Geometry check sheet. Reference: the model listing, model coordinates, mm. A direction names the side the tool comes from. Round coordinates to 2 decimals unless told otherwise and drop trailing zeros. Write item = value, one per line.
Autodesk Fusion 360 part; units mm, degrees
sketch "Sketch1" plane through (0, 0, 0) normal (0, 1, 0) x (1, 0, 0)
  circle A0 centre (0, 0) radius 3.3909
  circle A1 centre (0, 0) radius 2.3368
  dimension "d1" = 6.7818
  dimension "d2" = 4.6736
extrude "Extrude1" add sketch "Sketch1" along normal blind 1.9304
sketch "Sketch2" plane through (0, 1.9304, 0) normal (0, 1, 0) x (-1, 0, 0)
  circle A0 centre (0, 0) radius 2.3368
  circle A1 centre (0, 0) radius 3.3909
  line L0 (-10.0076, 10.0076) -> (10.0076, 10.0076) construction
  line L1 (10.0076, 10.0076) -> (10.0076, -10.0076) construction
  line L2 (10.0076, -10.0076) -> (-10.0076, -10.0076) construction
  line L3 (-10.0076, -10.0076) -> (-10.0076, 10.0076) construction
  line L4 (-10.0076, 10.0076) -> (10.0076, -10.0076) construction
  line L5 (10.0076, 10.0076) -> (-10.0076, -10.0076) construction
  circle A2 centre (7.9709, -7.9709) radius 2.0367 construction
  circle A3 centre (-7.9709, -7.9709) radius 2.0367 construction
  circle A4 centre (-7.9709, 7.9709) radius 2.0367 construction
  circle A5 centre (7.9709, 7.9709) radius 2.0367 construction
  circle A6 centre (0, 0) radius 5.334 construction
  circle A7 centre (7.9709, -7.9709) radius 0.5
  circle A8 centre (-7.9709, -7.9709) radius 0.5
  circle A9 centre (7.9709, 7.9709) radius 0.5
  circle A10 centre (-7.9709, 7.9709) radius 0.5
  line L6 (8.4709, -7.9709) -> (-8.4709, -7.9709) construction
  line L7 (0, -5.334) -> (0, 5.334) construction
  line L8 (5.334, 0) -> (-5.334, 0) construction
  line L9 (9.4111, -6.5307) -> (6.5307, -9.4111) construction
  line L10 (-6.5307, -9.4111) -> (-9.4111, -6.5307) construction
  line L11 (-9.4111, 6.5307) -> (-6.5307, 9.4111) construction
  line L12 (9.4111, 6.5307) -> (6.5307, 9.4111) construction
  line L13 (5.334, 0) -> (9.6916, -6.8813)
  line L14 (5.334, 0) -> (9.6916, 6.8813)
  line L15 (0, 5.334) -> (6.8813, 9.6916)
  line L16 (0, 5.334) -> (-6.8813, 9.6916)
  line L17 (-5.334, 0) -> (-9.6916, 6.8813)
  line L18 (-5.334, 0) -> (-9.6916, -6.8813)
  line L19 (0, -5.334) -> (-6.8813, -9.6916)
  line L20 (0, -5.334) -> (6.8813, -9.6916)
  arc A11 (6.8813, -9.6916) -> (9.6916, -6.8813) centre (7.9709, -7.9709) ccw
  arc A12 (-9.6916, -6.8813) -> (-6.8813, -9.6916) centre (-7.9709, -7.9709) ccw
  arc A13 (-6.8813, 9.6916) -> (-9.6916, 6.8813) centre (-7.9709, 7.9709) ccw
  arc A14 (9.6916, 6.8813) -> (6.8813, 9.6916) centre (7.9709, 7.9709) ccw
  circle A15 centre (0, 0) radius 1.143
  dimension "d5" = 20.0152
  dimension "d6" = 20.0152
  dimension "d7" = 10.668
  dimension "d8" = 1
  dimension "d9" = 16.9418
  dimension "d10" = 2.286
extrude "Extrude2" add sketch "Sketch2" along normal blind 1.651 contours A0 | A1 | A7 | A8 | A9 | A10 | L13 L14 L15 L16 L17 L18 L19 L20 A11 A12 A13 A14
sketch "Sketch3" plane through (0, 3.5814, 0) normal (0, 1, 0) x (-1, 0, 0)
  circle A0 centre (0, 0) radius 1.143
  line L0 (5.334, 0) -> (9.6916, 6.8813)
  arc A1 (9.6916, 6.8813) -> (6.8813, 9.6916) centre (7.9709, 7.9709) ccw
  line L1 (6.8813, 9.6916) -> (0, 5.334)
  line L2 (0, 5.334) -> (-6.8813, 9.6916)
  arc A2 (-6.8813, 9.6916) -> (-9.6916, 6.8813) centre (-7.9709, 7.9709) ccw
  line L3 (-9.6916, 6.8813) -> (-5.334, 0)
  line L4 (-5.334, 0) -> (-9.6916, -6.8813)
  arc A3 (-9.6916, -6.8813) -> (-6.8813, -9.6916) centre (-7.9709, -7.9709) ccw
  line L5 (-6.8813, -9.6916) -> (0, -5.334)
  line L6 (0, -5.334) -> (6.8813, -9.6916)
  arc A4 (6.8813, -9.6916) -> (9.6916, -6.8813) centre (7.9709, -7.9709) ccw
  line L7 (9.6916, -6.8813) -> (5.334, 0)
  line L8 (-10.0076, 10.0076) -> (10.0076, 10.0076) construction
  line L9 (10.0076, 10.0076) -> (10.0076, -10.0076) construction
  line L10 (10.0076, -10.0076) -> (-10.0076, -10.0076) construction
  line L11 (-10.0076, -10.0076) -> (-10.0076, 10.0076) construction
  line L12 (-10.0076, 10.0076) -> (10.0076, -10.0076) construction
  line L13 (10.0076, 10.0076) -> (-10.0076, -10.0076) construction
  line L14 (8.2888, -8.2888) -> (-8.2888, 8.2888) construction
  line L15 (-8.2888, -8.2888) -> (8.2888, 8.2888) construction
  line L16 (-8.4455, 8.4455) -> (8.4455, 8.4455) construction
  line L17 (8.4455, 8.4455) -> (8.4455, -8.4455) construction
  line L18 (8.4455, -8.4455) -> (-8.4455, -8.4455) construction
  line L19 (-8.4455, -8.4455) -> (-8.4455, 8.4455) construction
  line L20 (-8.4455, 8.4455) -> (8.4455, -8.4455) construction
  line L21 (8.4455, 8.4455) -> (-8.4455, -8.4455) construction
  circle A5 centre (7.9104, -7.9104) radius 0.5351
  circle A6 centre (-7.9104, -7.9104) radius 0.5351
  circle A7 centre (-7.9104, 7.9104) radius 0.5351
  circle A8 centre (7.9104, 7.9104) radius 0.5351
  line L22 (-6.376, 6.376) -> (6.376, 6.376) construction
  line L23 (6.376, 6.376) -> (6.376, -6.376) construction
  line L24 (6.376, -6.376) -> (-6.376, -6.376) construction
  line L25 (-6.376, -6.376) -> (-6.376, 6.376) construction
  line L26 (-6.376, 6.376) -> (6.376, -6.376) construction
  line L27 (6.376, 6.376) -> (-6.376, -6.376) construction
  line L28 (-6.5278, 6.5278) -> (6.5278, 6.5278) construction
  line L29 (6.5278, 6.5278) -> (6.5278, -6.5278) construction
  line L30 (6.5278, -6.5278) -> (-6.5278, -6.5278) construction
  line L31 (-6.5278, -6.5278) -> (-6.5278, 6.5278) construction
  line L32 (-6.5278, 6.5278) -> (6.5278, -6.5278) construction
  line L33 (6.5278, 6.5278) -> (-6.5278, -6.5278) construction
  circle A9 centre (6.0095, -6.0095) radius 0.5183
  circle A10 centre (-6.0095, -6.0095) radius 0.5183
  circle A11 centre (-6.0095, 6.0095) radius 0.5183
  circle A12 centre (6.0095, 6.0095) radius 0.5183
  line L34 (-4.826, -4.826) -> (4.826, -4.826) construction
  line L35 (4.826, -4.826) -> (4.826, 4.826) construction
  line L36 (4.826, 4.826) -> (-4.826, 4.826) construction
  line L37 (-4.826, 4.826) -> (-4.826, -4.826) construction
  line L38 (-4.826, -4.826) -> (4.826, 4.826) construction
  line L39 (4.826, -4.826) -> (-4.826, 4.826) construction
  line L40 (-4.6338, -4.6338) -> (4.6338, -4.6338) construction
  line L41 (4.6338, -4.6338) -> (4.6338, 4.6338) construction
  line L42 (4.6338, 4.6338) -> (-4.6338, 4.6338) construction
  line L43 (-4.6338, 4.6338) -> (-4.6338, -4.6338) construction
  line L44 (-4.6338, -4.6338) -> (4.6338, 4.6338) construction
  line L45 (4.6338, -4.6338) -> (-4.6338, 4.6338) construction
  circle A13 centre (4.1698, -4.1698) radius 0.6562
  circle A14 centre (-4.1698, -4.1698) radius 0.6562
  circle A15 centre (-4.1698, 4.1698) radius 0.6562
  circle A16 centre (4.1698, 4.1698) radius 0.6562
  dimension "d13" = 23.4442
  dimension "d14" = 16.891
  dimension "d15" = 16.891
  dimension "d16" = 18.034
  dimension "d17" = 13.0556
  dimension "d18" = 13.1064
  dimension "d19" = 9.652
hole "Hole1" at (-7.9104, 3.5814, -7.9104) at (-6.0095, 3.5814, -6.0095) at (-4.1698, 3.5814, -4.1698) at (-7.9104, 3.5814, 7.9104) at (-6.0095, 3.5814, 6.0095) at (-4.1698, 3.5814, 4.1698) at (7.9104, 3.5814, 7.9104) at (6.0095, 3.5814, 6.0095) at (4.1698, 3.5814, 4.1698) at (7.9104, 3.5814, -7.9104) at (6.0095, 3.5814, -6.0095) at (4.1698, 3.5814, -4.1698) direction (0, -1, 0) diameter 1 end through all
sketch "Sketch4" plane through (0, 3.5814, 0) normal (0, 1, 0) x (-1, 0, 0)
  circle A0 centre (-6.0095, -6.0095) radius 0.5
  circle A1 centre (-4.1698, 4.1698) radius 0.5
  circle A2 centre (-7.9104, 7.9104) radius 0.5
  circle A3 centre (6.0095, 6.0095) radius 0.5
  circle A4 centre (4.1698, -4.1698) radius 0.5
  circle A5 centre (7.9104, -7.9104) radius 0.5
  circle A6 centre (6.0095, -6.0095) radius 0.5
  circle A7 centre (7.9104, 7.9104) radius 0.5
  circle A8 centre (4.1698, 4.1698) radius 0.5
  circle A9 centre (-6.0095, 6.0095) radius 0.5
  circle A10 centre (-7.9104, -7.9104) radius 0.5
  circle A11 centre (-4.1698, -4.1698) radius 0.5
  circle A12 centre (0, 0) radius 1.143
  line L0 (5.334, 0) -> (9.6916, 6.8813)
  arc A13 (9.6916, 6.8813) -> (6.8813, 9.6916) centre (7.9709, 7.9709) ccw
  line L1 (6.8813, 9.6916) -> (0, 5.334)
  line L2 (0, 5.334) -> (-6.8813, 9.6916)
  arc A14 (-6.8813, 9.6916) -> (-9.6916, 6.8813) centre (-7.9709, 7.9709) ccw
  line L3 (-9.6916, 6.8813) -> (-5.334, 0)
  line L4 (-5.334, 0) -> (-9.6916, -6.8813)
  arc A15 (-9.6916, -6.8813) -> (-6.8813, -9.6916) centre (-7.9709, -7.9709) ccw
  line L5 (-6.8813, -9.6916) -> (0, -5.334)
  line L6 (0, -5.334) -> (6.8813, -9.6916)
  arc A16 (6.8813, -9.6916) -> (9.6916, -6.8813) centre (7.9709, -7.9709) ccw
  line L7 (9.6916, -6.8813) -> (5.334, 0)
  circle A17 centre (0, 0) radius 2.7305
  circle A18 centre (0, 0) radius 2.2098
  dimension "d22" = 5.461
  dimension "d23" = 4.4196
extrude "Extrude3" add sketch "Sketch4" along normal blind 0.508 contours A17
extrude "Extrude4" cut 1 faces at (-1.8417, 3.5814, -0.1666) along direction (0, -1, 0) blind 1.016 from surface at -0.508
extrude "Extrude5" cut 1 faces at (1.9259, 1.9304, 0.1729) along direction (0, 1, 0) blind 2.0066 from surface at -1.9304
(1) Scan lines: L1, parallel to Z at x = 6.25, y = 2.85; L2, parallel to Z at x = 8, y = 3.1; L3, parallel to Y at x = -4.5, z = -2.75. Record each from-to range of solid material in increasing order. Write a range as [from, to].
Answers follow:
L1 = [-9.29, -6.45], [-5.57, -1.45], [1.45, 5.57], [6.45, 9.29]
L2 = [-10.01, -8.4], [-7.42, -4.21], [4.21, 7.42], [8.4, 10.01]
L3 = [1.93, 3.58]
(2) Set-up check for faces 4 (the cylindrical face through (-5.71, 2.74, 5.61)), 5 (the flat face through (-3.39, 2.74, -7.48)), 6 (the flat face through (-1, 3.073, -1)): record each of +Z, -Z, +X, -X, +Y, -Y from which the full face is reachable in a straight line by a thin tool's end or side.
Answers follow:
face_4 = +Y, -Y
face_5 = -Z, +Y, -Y
face_6 = +Y
(3) Gauge pin test, flat ends, axial feed: pin 1 (1.8 mm diameter, centred on x = 0, z = 0, fed in from -Y); pin 2 (3 mm diameter, centred on x = 3.5, z = 4, fed in from -Y); pin 3 (2 mm diameter, centred on x = 0, z = -4.5, fed in from +Y). Record the tip position at first contact, or that the pin passes through.
Answers follow:
pin_1 = through
pin_2 = 1.93
pin_3 = 3.58
(4) Mould release check, pull along X, two halves, no side actions. Record for faces 1 (the flat face through (5, 1.93, 0)), 2 (the cylindrical face through (-2.604, 3.832, -0.82)), 3 (the cylindrical face through (9.44, 2.74, 9.38)): pulls with the +X half, pulls with the -X half, needs draft (parallel to the pull), parting line crosses it, or undercut.
Answers follow:
face_1 = needs draft
face_2 = parting line crosses it
face_3 = undercut
